Source: CAD feature listing. Evaluate the final solid. Frame: model axes, mm. Round coordinates to 2 decimals unless told otherwise and drop trailing zeros. Write each loop counter-clockwise with the first axis right and the second up, starting at its lowest first coordinate (ties: lowest second). Pieces come first, ordered by that corner, then holes. Notation, with made-up numbers: M 34,73 L 38,73 A26 ccw 38,89 Z; hole C 32.5,52.25 d8. An arc over 180 degrees is marked long. Use a Markdown table: item, result.
```python
from build123d import *

# Parameters (mm, degrees)
SKETCH1_R           = 1
SKETCH1_R_2         = 0.999999999
SKETCH1_R_3         = 1.000000001
SKETCH1_R_4         = 1.000000003
SKETCH1_R_5         = 0.999999997
BOSS_EXTRUDE1_DEPTH = 3
SKETCH2_W           = 6.5
SKETCH2_H           = 3.5
CUT_EXTRUDE1_DEPTH  = 3


with BuildPart() as part:
    # Sketch1 → Boss-Extrude1 (new body)
    with BuildSketch(Plane(origin=(0, 0, 0), x_dir=(1, 0, 0), z_dir=(0, 1, 0))):
        with BuildLine():
            Line((-65.541413555, 48.16007559), (-33.218669872, 45.046086874))
            ThreePointArc((-33.218669872, 45.046086874), (-32.739740879, 45.011528364), (-32.25970508, 45))
            Line((-32.25970508, 45), (32.25970508, 45))
            ThreePointArc((32.25970508, 45), (32.739740879, 45.011528364), (33.218669872, 45.046086874))
            Line((33.218669872, 45.046086874), (65.541413555, 48.16007559))
            ThreePointArc((65.541413555, 48.16007559), (68.051615849, 48.735029299), (70.331753828, 49.931966272))
            ThreePointArc((70.331753828, 49.931966272), (81.716587017, 44.695249474), (71.540883348, 37.381380156))
            ThreePointArc((71.540883348, 37.381380156), (69.074176187, 38.121003778), (66.500378347, 38.206162463))
            Line((66.500378347, 38.206162463), (37.020517604, 35.366058461))
            ThreePointArc((37.020517604, 35.366058461), (34.967820887, 34.700490182), (33.386772404, 33.231874971))
            ThreePointArc((33.386772404, 33.231874971), (34.463229219, 29.741424145), (35.835420758, 26.3562954))
            ThreePointArc((35.835420758, 26.3562954), (35.77253489, 25.409347753), (34.946904251, 24.941374967))
            ThreePointArc((34.946904251, 24.941374967), (33.213559493, 24.190832889), (32.5, 22.441938863))
            Line((32.5, 22.441938863), (32.5, -22.441938863))
            ThreePointArc((32.5, -22.441938863), (33.213559493, -24.190832889), (34.946904251, -24.941374967))
            ThreePointArc((34.946904251, -24.941374967), (35.77253489, -25.409347753), (35.835420758, -26.3562954))
            ThreePointArc((35.835420758, -26.3562954), (34.463229219, -29.741424145), (33.386772404, -33.231874971))
            ThreePointArc((33.386772404, -33.231874971), (34.967820887, -34.700490182), (37.020517604, -35.366058461))
            Line((37.020517604, -35.366058461), (66.500378347, -38.206162463))
            ThreePointArc((66.500378347, -38.206162463), (69.074176187, -38.121003778), (71.540883348, -37.381380156))
            ThreePointArc((71.540883348, -37.381380156), (81.716587017, -44.695249474), (70.331753828, -49.931966272))
            ThreePointArc((70.331753828, -49.931966272), (68.051615849, -48.735029299), (65.541413555, -48.16007559))
            Line((65.541413555, -48.16007559), (33.218669872, -45.046086874))
            ThreePointArc((33.218669872, -45.046086874), (32.739740879, -45.011528364), (32.25970508, -45))
            Line((32.25970508, -45), (-32.25970508, -45))
            ThreePointArc((-32.25970508, -45), (-32.739740879, -45.011528364), (-33.218669872, -45.046086874))
            Line((-33.218669872, -45.046086874), (-65.541413555, -48.16007559))
            ThreePointArc((-65.541413555, -48.16007559), (-68.051615849, -48.735029299), (-70.331753828, -49.931966272))
            ThreePointArc((-70.331753828, -49.931966272), (-81.716587017, -44.695249474), (-71.540883348, -37.381380156))
            ThreePointArc((-71.540883348, -37.381380156), (-69.074176187, -38.121003778), (-66.500378347, -38.206162463))
            Line((-66.500378347, -38.206162463), (-37.020517604, -35.366058461))
            ThreePointArc((-37.020517604, -35.366058461), (-34.967820887, -34.700490182), (-33.386772404, -33.231874971))
            ThreePointArc((-33.386772404, -33.231874971), (-34.463229219, -29.741424145), (-35.835420758, -26.3562954))
            ThreePointArc((-35.835420758, -26.3562954), (-35.77253489, -25.409347753), (-34.946904251, -24.941374967))
            ThreePointArc((-34.946904251, -24.941374967), (-33.213559493, -24.190832889), (-32.5, -22.441938863))
            Line((-32.5, -22.441938863), (-32.5, 22.441938863))
            ThreePointArc((-32.5, 22.441938863), (-33.213559493, 24.190832889), (-34.946904251, 24.941374967))
            ThreePointArc((-34.946904251, 24.941374967), (-35.77253489, 25.409347753), (-35.835420758, 26.3562954))
            ThreePointArc((-35.835420758, 26.3562954), (-34.463229219, 29.741424145), (-33.386772404, 33.231874971))
            ThreePointArc((-33.386772404, 33.231874971), (-34.967820887, 34.700490182), (-37.020517604, 35.366058461))
            Line((-37.020517604, 35.366058461), (-66.500378347, 38.206162463))
            ThreePointArc((-66.500378347, 38.206162463), (-69.074176187, 38.121003778), (-71.540883348, 37.381380156))
            ThreePointArc((-71.540883348, 37.381380156), (-81.716587017, 44.695249474), (-70.331753828, 49.931966272))
            ThreePointArc((-70.331753828, 49.931966272), (-68.051615849, 48.735029299), (-65.541413555, 48.16007559))
        make_face()
        with Locations(Location((-79, 44, 0), (0, 0, 270))):
            Circle(SKETCH1_R, mode=Mode.SUBTRACT)
        with Locations(Location((79, -44, 0), (0, 0, 270))):
            Circle(SKETCH1_R, mode=Mode.SUBTRACT)
        with Locations(Location((79, 44, 0), (0, 0, 270))):
            Circle(SKETCH1_R, mode=Mode.SUBTRACT)
        with Locations(Location((-74.500002545, 48.500002545, 0), (0, 0, 270))):
            Circle(SKETCH1_R_2, mode=Mode.SUBTRACT)
        with Locations(Location((-70, 44.00000509, 0), (0, 0, 270))):
            Circle(SKETCH1_R_3, mode=Mode.SUBTRACT)
        with Locations(Location((-74.499997455, 39.500002545, 0), (0, 0, 270))):
            Circle(SKETCH1_R_4, mode=Mode.SUBTRACT)
        with Locations(Location((-74.499997455, -39.500002545, 0), (0, 0, 270))):
            Circle(SKETCH1_R_3, mode=Mode.SUBTRACT)
        with Locations(Location((-70, -44.00000509, 0), (0, 0, 270))):
            Circle(SKETCH1_R_2, mode=Mode.SUBTRACT)
        with Locations(Location((-74.500002545, -48.500002545, 0), (0, 0, 270))):
            Circle(SKETCH1_R_5, mode=Mode.SUBTRACT)
        with Locations(Location((-79, -44, 0), (0, 0, 270))):
            Circle(SKETCH1_R, mode=Mode.SUBTRACT)
        with Locations(Location((74.500002545, -48.500002545, 0), (0, 0, 270))):
            Circle(SKETCH1_R_3, mode=Mode.SUBTRACT)
        with Locations(Location((70, -44.00000509, 0), (0, 0, 270))):
            Circle(SKETCH1_R_2, mode=Mode.SUBTRACT)
        with Locations(Location((74.499997455, -39.500002545, 0), (0, 0, 270))):
            Circle(SKETCH1_R_5, mode=Mode.SUBTRACT)
        with Locations(Location((74.499997455, 39.500002545, 0), (0, 0, 270))):
            Circle(SKETCH1_R_2, mode=Mode.SUBTRACT)
        with Locations(Location((70, 44.00000509, 0), (0, 0, 270))):
            Circle(SKETCH1_R_3, mode=Mode.SUBTRACT)
        with Locations(Location((74.500002545, 48.500002545, 0), (0, 0, 270))):
            Circle(SKETCH1_R_4, mode=Mode.SUBTRACT)
        with Locations(Location((-74.5, -44, 0), (0, 0, 270))):
            Circle(SKETCH1_R, mode=Mode.SUBTRACT)
        with Locations(Location((-74.5, 44, 0), (0, 0, 270))):
            Circle(SKETCH1_R, mode=Mode.SUBTRACT)
        with Locations(Location((74.5, 44, 0), (0, 0, 270))):
            Circle(SKETCH1_R, mode=Mode.SUBTRACT)
        with Locations(Location((74.5, -44, 0), (0, 0, 270))):
            Circle(SKETCH1_R, mode=Mode.SUBTRACT)
    extrude(amount=BOSS_EXTRUDE1_DEPTH)

    # Sketch2 → Cut-Extrude1 (cut)
    with BuildSketch(Plane(origin=(0, 3, 0), x_dir=(1, 0, 0), z_dir=(0, 1, 0))):
        with Locations((-17.75, 23.75)):
            Rectangle(SKETCH2_W, SKETCH2_H)
        with Locations((-17.75, -23.75)):
            Rectangle(SKETCH2_W, SKETCH2_H)
        with Locations((17.75, -23.75)):
            Rectangle(SKETCH2_W, SKETCH2_H)
        with Locations((17.75, 23.75)):
            Rectangle(SKETCH2_W, SKETCH2_H)
        with BuildLine():
            Line((-25.5, 19), (-4, 19))
            ThreePointArc((-4, 19), (-3.292893219, 18.707106781), (-3, 18))
            Line((-3, 18), (-3, 2.5))
            ThreePointArc((-3, 2.5), (-3.292893219, 1.792893219), (-4, 1.5))
            Line((-4, 1.5), (-25.5, 1.5))
            ThreePointArc((-25.5, 1.5), (-26.207106781, 1.792893219), (-26.5, 2.5))
            Line((-26.5, 2.5), (-26.5, 18))
            ThreePointArc((-26.5, 18), (-26.207106781, 18.707106781), (-25.5, 19))
        make_face()
        with BuildLine():
            Line((-25.5, -1.5), (-4, -1.5))
            ThreePointArc((-4, -1.5), (-3.292893219, -1.792893219), (-3, -2.5))
            Line((-3, -2.5), (-3, -18))
            ThreePointArc((-3, -18), (-3.292893219, -18.707106781), (-4, -19))
            Line((-4, -19), (-25.5, -19))
            ThreePointArc((-25.5, -19), (-26.207106781, -18.707106781), (-26.5, -18))
            Line((-26.5, -18), (-26.5, -2.5))
            ThreePointArc((-26.5, -2.5), (-26.207106781, -1.792893219), (-25.5, -1.5))
        make_face()
        with BuildLine():
            Line((4, 19), (25.5, 19))
            ThreePointArc((25.5, 19), (26.207106781, 18.707106781), (26.5, 18))
            Line((26.5, 18), (26.5, 2.5))
            ThreePointArc((26.5, 2.5), (26.207106781, 1.792893219), (25.5, 1.5))
            Line((25.5, 1.5), (4, 1.5))
            ThreePointArc((4, 1.5), (3.292893219, 1.792893219), (3, 2.5))
            Line((3, 2.5), (3, 18))
            ThreePointArc((3, 18), (3.292893219, 18.707106781), (4, 19))
        make_face()
        with BuildLine():
            Line((4, -1.5), (25.5, -1.5))
            ThreePointArc((25.5, -1.5), (26.207106781, -1.792893219), (26.5, -2.5))
            Line((26.5, -2.5), (26.5, -18))
            ThreePointArc((26.5, -18), (26.207106781, -18.707106781), (25.5, -19))
            Line((25.5, -19), (4, -19))
            ThreePointArc((4, -19), (3.292893219, -18.707106781), (3, -18))
            Line((3, -18), (3, -2.5))
            ThreePointArc((3, -2.5), (3.292893219, -1.792893219), (4, -1.5))
        make_face()
        with BuildLine():
            Line((-17.595187003, 39), (17.595187003, 39))
            ThreePointArc((17.595187003, 39), (18.554660419, 38.281799152), (18.135944594, 37.158821525))
            Line((18.135944594, 37.158821525), (0.540757591, 25.84762988))
            ThreePointArc((0.540757591, 25.84762988), (0, 25.688808356), (-0.540757591, 25.84762988))
            Line((-0.540757591, 25.84762988), (-18.135944594, 37.158821525))
            ThreePointArc((-18.135944594, 37.158821525), (-18.554660419, 38.281799152), (-17.595187003, 39))
        make_face()
        with BuildLine():
            Line((-17.595187003, -39), (17.595187003, -39))
            ThreePointArc((17.595187003, -39), (18.554660419, -38.281799152), (18.135944594, -37.158821525))
            Line((18.135944594, -37.158821525), (0.540757591, -25.84762988))
            ThreePointArc((0.540757591, -25.84762988), (0, -25.688808356), (-0.540757591, -25.84762988))
            Line((-0.540757591, -25.84762988), (-18.135944594, -37.158821525))
            ThreePointArc((-18.135944594, -37.158821525), (-18.554660419, -38.281799152), (-17.595187003, -39))
        make_face()
    extrude(amount=-CUT_EXTRUDE1_DEPTH, mode=Mode.SUBTRACT)


solid = part.part
```
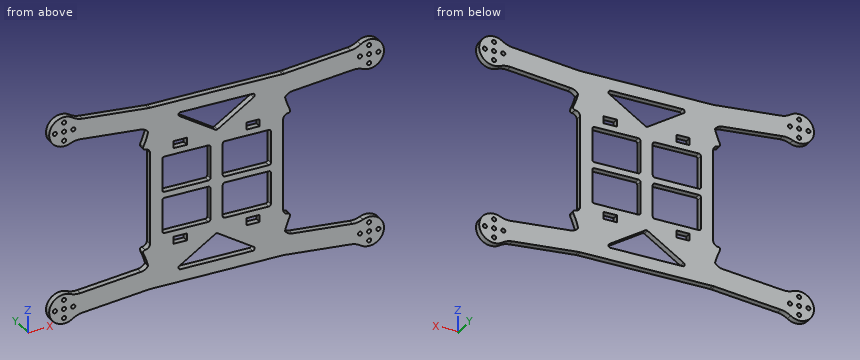
Q1. Section D-D on y = 0.9. Give the number of separate pieces and of enclosed holes in the cut face, plus the area to 3 significant figures.
Results are:
| item | result |
|---|---|
| separate pieces | 1 |
| enclosed holes | 30 |
| area | 5,680 mm^2 |
Q2. Section B-B on x = 57. Return loops of the section in (y, z).
Results are:
| item | result |
|---|---|
| outline | M 0,-47.34 L 3,-47.34 L 3,-37.29 L 0,-37.29 Z; M 0,37.29 L 3,37.29 L 3,47.34 L 0,47.34 Z |
Q3. Section A-A on z = -11.5. Return loops of the section in (x, y).
Results are:
| item | result |
|---|---|
| outline | M -32.5,0 L -26.5,0 L -26.5,3 L -32.5,3 Z; M -3,0 L 3,0 L 3,3 L -3,3 Z; M 26.5,0 L 32.5,0 L 32.5,3 L 26.5,3 Z |
Q4. Section C-C on z = 30. Return loops of the section in (x, y).
Results are:
| item | result |
|---|---|
| outline | M -34.37,0 L -7,0 L -7,3 L -34.37,3 Z; M 7,0 L 34.37,0 L 34.37,3 L 7,3 Z |
Q5. First-contact query: pin 1 Ø0.9 at (x, y) = (17.5, 2) entering from +Z; pin 2 Ø2.5 at (x, z) = (-74.5, -48.5) entering from -Y; pin 3 Ø0.9 at (y, z) = (1.5, 23.5) entering from -X; pin 4 Ø0.9 at (y, z) = (1.5, 23.5) entering from +X. Flat tips, straight axial feed; report the tip coordinate or a pass-through.
Results are:
| item | result |
|---|---|
| pin 1 | z = 45 |
| pin 2 | y = 0 |
| pin 3 | x = -33.01 |
| pin 4 | x = 33.01 |
Q6. Line query: L1, parallel to X at y = 1.5, z = 16.5; L2, parallel to Z at x = -1.5, y = 0.2; L3, parallel to X at y = 0.6, z = -39.5. Output: solid intervals per line, ascending.
Results are:
| item | result |
|---|---|
| L1 | -32.5 to -26.5, -3 to 3, 26.5 to 32.5 |
| L2 | -45 to -39, -26.46 to 26.46, 39 to 45 |
| L3 | -80.18 to -75.5, -73.5 to 73.5, 75.5 to 80.18 |
